from build123d import *

# Parameters (mm, degrees)
F0_W     = 1143
F0_H     = 76.2
F1_DEPTH = 19.05
F2_W     = 50.8
F2_H     = 19.05
F3_DEPTH = 19.05
F4_R     = 9.525
F5_DEPTH = 19.05
F6_W     = 22.86
F6_H     = 15.875
F7_DEPTH = 25.4
F9_DEPTH = 25.4


# Not quite as in the source:
# - a length typed as a fraction of an inch, garbled in the dataset ("3 / 203.2 mm" for 3/8 in), is restored
# - a feature names something its author has since deleted; it is built from what else it names


with BuildPart() as f1:
    # F0 (on Top) → F1 (new body)
    with BuildSketch(Plane.XY):
        with Locations((571.5, -38.1)):
            Rectangle(F0_W, F0_H)
    extrude(amount=F1_DEPTH)

    # F2 (on face) → F3 (join)
    with BuildSketch(Plane(origin=(0, 0, 0), x_dir=(-1, 0, 0), z_dir=(0, 1, 0))):
        with Locations((-927.1, 9.525)):
            Rectangle(F2_W, F2_H)
        with Locations((-749.3, 9.525)):
            Rectangle(F2_W, F2_H)
        with Locations((-571.5, 9.525)):
            Rectangle(F2_W, F2_H)
        with Locations((-393.7, 9.525)):
            Rectangle(F2_W, F2_H)
        with Locations((-215.9, 9.525)):
            Rectangle(F2_W, F2_H)
    extrude(amount=F3_DEPTH)

    # F4 (on face) → F5 (cut)
    with BuildSketch(Plane.XY.offset(19.05)):
        with Locations((143.6968424, -38.1)):
            Circle(F4_R)
    extrude(amount=-F5_DEPTH, mode=Mode.SUBTRACT)

    # F6 (on face) → F7 (cut)
    with BuildSketch(Plane.XY.offset(19.05)):
        with Locations((1047.75, -7.9375)):
            Rectangle(F6_W, F6_H)
    extrude(amount=-F7_DEPTH, mode=Mode.SUBTRACT)

    # F8 (on face) → F9 (cut)
    with BuildSketch(Plane.XY.offset(19.05)):
        Polygon((1036.32, 0), (966.4863944054, 0), (966.4863944054, -76.2), (1143, -76.2), (1143, 0), (1059.18, 0), (1059.18, -15.875), (1036.32, -15.875), align=None)
    extrude(amount=-F9_DEPTH, mode=Mode.SUBTRACT)


solid = f1.part
The listing builds one solid part. Answer for the finished solid, in the listing's coordinates (mm). A direction names the side the tool comes from. Coordinates: 2 decimals unless noted, no trailing zeros. Loops run counter-clockwise (first coordinate to the right, second up) from the corner with the lowest first, then second, coordinate; pieces in that order, holes last. Notation, with made-up numbers: (-16.75, 60.25) -> (0.25, 60.25) arc R14 ccw to (0.25, 78.25) -> close; hole circle Ø10 at (-34, 42). An arc over 180 degrees is marked (long way). Answer in a Markdown table with one row per item. Add a question column.
1. The part is cut by section B-B, the plane z = 12.25. Write down the section's boundary in (x, y) (3 decimals).
2. For faces 5 (the flat face through (94, 0, 9)), 6 (the flat face through (572, 19.05, 10)), 7 (the flat face through (952.5, 9, 9)), 8 (the flat face through (304, 0, 9)), determine the directions among +Z, -Z, +X, -X, +Y, -Y from which every point of the face is accessible in a straight line to the end or side of a thin tool.
3. The part is cut by section A-A, the plane y = -38.1. Write down the section's boundary in (x, z).
4. Consider line 1 (X direction, y = 15.5, z = 13.25); line 2 (Y direction, x = 500.5, z = 8); line 3 (Y direction, x = 151.5, z = 5.75). Determine where each line is inside the solid, lowest interval first. Write a range as [from, to].
5. Flat-ended cylindrical pins translate along their axes: P1, Ø2, axis at y = -54.5, z = 2, coming from the -X side; P2, Ø5.5, axis at x = 685.5, z = 7, coming from the +Y side; P3, Ø15, axis at x = 143.7, y = -38.1, coming from the +Z side; P4, Ø10, axis at y = 9, z = 2.5, coming from the +X side. Find the tip coordinate at first contact, or state that the pin passes through.
6. Determine the mould class of faces 1 (the flat face through (966.486, -38, 10)), 2 (the flat face through (476, -38, 0)), 3 (the flat face through (546.1, 9, 9)), 4 (the flat face through (0, -39, 9)) for opening direction X: +X half, -X half, draft (parallel to the pull), parting line (faces both ways), or undercut.
7. The part is cut by section C-C, the plane x = 85.5. Write down the section's boundary in (y, z).
Answer below:
| question | item | result |
|---|---|---|
| 1 | outline | (0, -76.2) -> (966.486, -76.2) -> (966.486, 0) -> (952.5, 0) -> (952.5, 19.05) -> (901.7, 19.05) -> (901.7, 0) -> (774.7, 0) -> (774.7, 19.05) -> (723.9, 19.05) -> (723.9, 0) -> (596.9, 0) -> (596.9, 19.05) -> (546.1, 19.05) -> (546.1, 0) -> (419.1, 0) -> (419.1, 19.05) -> (368.3, 19.05) -> (368.3, 0) -> (241.3, 0) -> (241.3, 19.05) -> (190.5, 19.05) -> (190.5, 0) -> (0, 0) -> close; hole circle Ø19.05 at (143.697, -38.1) |
| 2 | face 5 | +Z, -Z, -X, +Y |
| 2 | face 6 | +Z, -Z, +X, -X, +Y |
| 2 | face 7 | +Z, -Z, +X, +Y |
| 2 | face 8 | +Z, -Z, +Y |
| 3 | outline | (0, 0) -> (134.17, 0) -> (134.17, 19.05) -> (0, 19.05) -> close; (153.22, 0) -> (966.49, 0) -> (966.49, 19.05) -> (153.22, 19.05) -> close |
| 4 | line 1 | [190.5, 241.3], [368.3, 419.1], [546.1, 596.9], [723.9, 774.7], [901.7, 952.5] |
| 4 | line 2 | [-76.2, 0] |
| 4 | line 3 | [-76.2, -43.56], [-32.64, 0] |
| 5 | P1 | x = 0 |
| 5 | P2 | y = 0 |
| 5 | P3 | through |
| 5 | P4 | x = 952.5 |
| 6 | face 1 | +X half |
| 6 | face 2 | draft |
| 6 | face 3 | undercut |
| 6 | face 4 | -X half |
| 7 | outline | (-76.2, 0) -> (0, 0) -> (0, 19.05) -> (-76.2, 19.05) -> close |
